Design review of the part built by this model. Coordinates are the model's own, in mm. Face numbers are marked on the shaded views. A direction names the side the tool comes from. Round coordinates to 2 decimals unless told otherwise and drop trailing zeros. Order: outer loops, then holes, each group sorted by start corner. A loop starts at its lowest first (then second) coordinate and runs counter-clockwise, first axis right, second up. Notation, with made-up numbers: (53.5, 24.5) - (76.5, 24.5) arc R22 ccw to (76.5, 52.5) - close; hole circle Ø9 at (77.25, 64.5). An arc over 180 degrees is marked (long way). Write item = value, one per line.
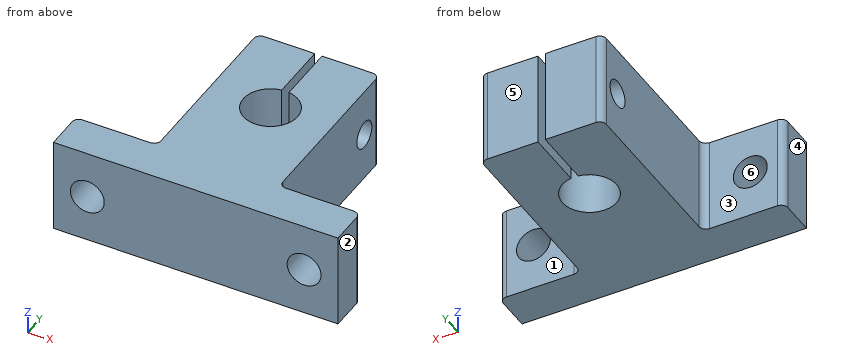
from build123d import *

# Parameters (mm, degrees)
SKETCH_1_R          = 4
EXTRUDE_1_DEPTH     = 14
SKETCH_2_R          = 2.5
CUT_EXTRUDE_1_DEPTH = 14
SKETCH_3_W          = 1.071241762
SKETCH_3_H          = 14
CUT_EXTRUDE_2_DEPTH = 14
SKETCH_4_R          = 2
CUT_EXTRUDE_3_DEPTH = 60
FILLET_1_R          = 1
FILLET_2_R          = 1


with BuildPart() as part:
    # 草图1 → 凸台-拉伸1 (new body)
    with BuildSketch(Plane.XY):
        Polygon((-22.707070707, -12.272727273), (19.292929293, -12.272727273), (19.292929293, -6.272727273), (7.292929293, -6.272727273), (7.292929293, 20.527272727), (0.929292929, 20.527272727), (-10.707070707, 20.527272727), (-10.707070707, -6.272727273), (-22.707070707, -6.272727273), align=None)
        with Locations((-1.707070707, 7.727272727)):
            Circle(SKETCH_1_R, mode=Mode.SUBTRACT)
    extrude(amount=EXTRUDE_1_DEPTH)

    # 草图2 → 切除-拉伸1 (cut)
    with BuildSketch(Plane(origin=(0, -6.272727273, 0), x_dir=(1, 0, 0), z_dir=(0, 1, 0))):
        with Locations((-17.707070707, -7)):
            Circle(SKETCH_2_R)
        with Locations((14.292929293, -7)):
            Circle(SKETCH_2_R)
    extrude(amount=-CUT_EXTRUDE_1_DEPTH, mode=Mode.SUBTRACT)

    # 草图3 → 切除-拉伸2 (cut)
    with BuildSketch(Plane(origin=(0, 20.527272727, 0), x_dir=(1, 0, 0), z_dir=(0, 1, 0))):
        with Locations((-1.707070707, -7)):
            Rectangle(SKETCH_3_W, SKETCH_3_H)
    extrude(amount=-CUT_EXTRUDE_2_DEPTH, mode=Mode.SUBTRACT)

    # 草图4 → 切除-拉伸3 (cut)
    with BuildSketch(Plane(origin=(7.292929293, 0, 0), x_dir=(0, 0, -1), z_dir=(1, 0, 0))):
        with Locations((-7, 16.527272727)):
            Circle(SKETCH_4_R)
    extrude(amount=-CUT_EXTRUDE_3_DEPTH, mode=Mode.SUBTRACT)

    # 圆角1
    fillet_1_edges = [part.edges().sort_by_distance(p)[0] for p in [
        (7.292929293, 20.527272727, 7),
        (19.292929293, -6.272727273, 7),
        (-22.707070707, -6.272727273, 7),
        (-10.707070707, 20.527272727, 7),
    ]]
    fillet(fillet_1_edges, radius=FILLET_1_R)

    # 圆角2
    fillet_2_edges = [part.edges().sort_by_distance(p)[0] for p in [
        (7.292929293, -6.272727273, 7),
        (-10.707070707, -6.272727273, 7),
    ]]
    fillet(fillet_2_edges, radius=FILLET_2_R)


solid = part.part
Item 1: Insertion check: P1, Ø2.5, axis at y = 18, z = 10, coming from the -X side; P2, Ø4, axis at y = 11.5, z = 9, coming from the +X side; P3, Ø5, axis at x = 11, z = 7, coming from the +Y side. Each pin has a flat end and moves straight along its axis. Give the tip position at first contact, or say it passes through.
Data:
P1 = -10.71
P2 = 7.29
P3 = -6.27
Item 2: Take a section at B-B, the plane x = -18. State the section outline as (y, z) points.
Data:
outline = (-12.27, 0) - (-6.27, 0) - (-6.27, 4.52) - (-12.27, 4.52) - close; (-12.27, 9.48) - (-6.27, 9.48) - (-6.27, 14) - (-12.27, 14) - close
Item 3: Take a section at C-C, the plane y = -9. State the section outline as (x, z) points.
Data:
outline = (-22.71, 0) - (19.29, 0) - (19.29, 14) - (-22.71, 14) - close; hole circle Ø5 at (-17.71, 7); hole circle Ø5 at (14.29, 7)
Item 4: For line 1 along X through (y, z) = (-10.5, 7); line 2 along X through (y, z) = (14.5, 1.5); line 3 along Y through (x, z) = (0.5, 6.5), list the stretches that pass through material, from the lowest coordinate up. Write a range as [from, to].
Data:
line_1 = [-22.71, -20.21], [-15.21, 11.79], [16.79, 19.29]
line_2 = [-10.71, -2.24], [-1.17, 7.29]
line_3 = [-12.27, 4.39], [11.06, 14.59], [18.46, 20.53]
Item 5: The part is to be moulded in two halves that separate along X. For the marked faces 4, 5 and 6, say which applies: +X half, -X half, draft (parallel to the pull), parting line (faces both ways), or undercut.
Data:
face_4 = -X half
face_5 = draft
face_6 = undercut
Item 6: For the marked faces 1, 2 and 3, list the 3-axis set-ups (+Z, -Z, +X, -X, +Y, -Y) from which the entire face can be reached by the end or side of a thin tool; tool diameter is ignored.
Data:
face_1 = +Z, -Z, +X, +Y
face_2 = +Z, -Z, +X, +Y, -Y
face_3 = +Z, -Z, -X, +Y
Item 7: Take a section at D-D, the plane z = 10. State the section outline as (x, y) points, and give its area (3 significant figures).
Data:
outline = (-22.71, -12.27) - (19.29, -12.27) - (19.29, -7.27) arc R1 ccw to (18.29, -6.27) - (8.29, -6.27) arc R1 cw to (7.29, -5.27) - (7.29, 19.53) arc R1 ccw to (6.29, 20.53) - (-1.17, 20.53) - (-1.17, 11.69) arc R4 cw (long way) to (-2.24, 11.69) - (-2.24, 20.53) - (-9.71, 20.53) arc R1 ccw to (-10.71, 19.53) - (-10.71, -5.27) arc R1 cw to (-11.71, -6.27) - (-21.71, -6.27) arc R1 ccw to (-22.71, -7.27) - close
area = 674 mm2
Item 8: Take a section at A-A, the plane z = 7. Count the separate pieces of the cut face and the enclosed holes in it, and give its area (3 significant figures).
Data:
separate_pieces = 5
enclosed_holes = 0
area = 547 mm2
